Read the model definition and answer for the solid it produces. Units are mm, in the model's axes. A direction names the side the tool comes from. Round coordinates to 2 decimals unless told otherwise and drop trailing zeros. Order: outer loops, then holes, each group sorted by start corner. A loop starts at its lowest first (then second) coordinate and runs counter-clockwise, first axis right, second up. Notation, with made-up numbers: (11.25, 30.25) -> (52.25, 30.25) arc R32 cw to (52.25, 58.25) -> close; hole circle Ø11 at (18.25, 66.25). An arc over 180 degrees is marked (long way). Answer as a JSON object with one key per item and string values. Group by question number.
Item 1: Section B-B, the plane y = 26 is taken. Write down the section's boundary in (x, z), plus the area to 3 significant figures.
Item 2: Consider probe 1 along X at (y, z) = (96, 0); probe 2 along Z at (x, y) = (16, 57); probe 3 along X at (y, z) = (99, 0) (3 decimals). Determine where each line is inside the solid, lowest interval first. Write a range as from..to.
Item 3: Section C-C, the plane y = 7 is taken. Write down the section's boundary in (x, z) (3 decimals).
Item 4: Given P1, Ø5, axis at x = 8, y = 11, coming from the +Z side; P2, Ø1.3, axis at x = -11.5, y = 99, coming from the +Z side; P3, Ø0.6, axis at x = -11.5, z = 0, coming from the -Y side, each flat-ended and moving along its own axis, determine where each tip first touches the part or whether it passes through.
Item 5: The mould has two halves that part along Y. Classify faces 1 (the flat face through (5, 100, 10)), 2 (the flat face through (0, 92.5, 0)), 3 (the flat face through (-12, 99, 0)): pulls with the +Y half, pulls with the -Y half, needs draft (parallel to the pull), parting line crosses it, or undercut.
Item 6: For faces 4 (the flat face through (18.5, 0, 20.6)), 5 (the cylindrical face through (-10.74, 97.54, -2.38)), 6 (the cylindrical face through (-12.258, 93.079, -0.418)), determine the directions among +Z, -Z, +X, -X, +Y, -Y from which every point of the face is accessible in a straight line to the end or side of a thin tool.
Item 7: Section A-A, the plane x = 0 is taken. Write down the section's boundary in (y, z), plus the area to 3 significant figures.
from build123d import *

# Parameters (mm, degrees)
SKETCH2_R          = 12.5
SKETCH1_R          = 30
SKETCH5_R          = 11
CUT_EXTRUDE2_DEPTH = 5
SKETCH7_W          = 4
SKETCH7_H          = 3
CUT_EXTRUDE4_DEPTH = 12
SKETCH8_R          = 1
CUT_EXTRUDE6_DEPTH = 106.854123131
CHAMFER1_SIZE      = 2
CHAMFER1_SIZE2     = 2.698735062


# Read off the part's stored shape, not the designer's step: Shell2
with BuildPart() as part:
    # Sketch2 → Loft1 section 0
    with BuildSketch(Plane(origin=(0, 100, 0), x_dir=(1, 0, 0), z_dir=(0, 1, 0))):
        Circle(SKETCH2_R)
    # Sketch1 → Loft1 section 1
    with BuildSketch(Plane(origin=(0, 0, 0), x_dir=(1, 0, 0), z_dir=(0, 1, 0))):
        Circle(SKETCH1_R)
    loft()

    # Sketch5 → Cut-Extrude2 (cut)
    with BuildSketch(Plane(origin=(0, 100, 0), x_dir=(1, 0, 0), z_dir=(0, 1, 0))):
        with Locations(Location((0, 0, 0), (0, 0, 270))):
            Circle(SKETCH5_R)
    extrude(amount=-CUT_EXTRUDE2_DEPTH, mode=Mode.SUBTRACT)

    # Sketch7 → Cut-Extrude4 (cut)
    with BuildSketch(Plane(origin=(0, 0, 0), x_dir=(0, 0, -1), z_dir=(1, 0, 0))):
        with Locations((-0.000948901, 98.479870862)):
            Rectangle(SKETCH7_W, SKETCH7_H)
    extrude(amount=-CUT_EXTRUDE4_DEPTH, mode=Mode.SUBTRACT)

    # Shell2 outline → Shell2 (revolve, cut)
    with BuildSketch(Plane.XY):
        Polygon((11.274507437, 92.5), (0, 92.5), (0, 0), (27.462007437, 0), align=None)
    revolve(axis=Axis((0, 0, 0), (0, 1, 0)), mode=Mode.SUBTRACT)

    # Sketch8 → Cut-Extrude6 (cut, through all)
    with BuildSketch(Plane(origin=(0, 96.979870862, 0), x_dir=(1, 0, 0), z_dir=(0, 1, 0))):
        with Locations(Location((-11.275969927, 0.228612613, 0), (0, 0, 271.596209632))):
            Circle(SKETCH8_R)
    extrude(amount=-CUT_EXTRUDE6_DEPTH, mode=Mode.SUBTRACT)

    # Chamfer1
    chamfer1_edges = [part.edges().sort_by_distance(p)[0] for p in [
        (-30, 0, 0),
    ]]
    chamfer1_side = [part.faces().sort_by_distance(p)[0] for p in [
        (-29.151471863, 0, 0),
    ]]
    chamfer(chamfer1_edges, length=CHAMFER1_SIZE, length2=CHAMFER1_SIZE2, reference=chamfer1_side[0])


solid = part.part
Values found:
{
 "1": {"outline": "circle Ø50.9 at (0, 0); hole circle Ø45.82 at (0, 0)", "area": "386 mm2"},
 "2": {"probe 1": "-13.2..-12.25, 11..13.2", "probe 2": "-12.04..-7.06, 7.06..12.04", "probe 3": "-12.675..-12, 11..12.675"},
 "3": {"outline": "circle Ø57.55 at (0, 0); hole circle Ø52.474 at (0, 0)"},
 "4": {"P1": "z = 27.7", "P2": "z = 6.57", "P3": "y = 99.98"},
 "5": {"face 1": "pulls with the +Y half", "face 2": "pulls with the -Y half", "face 3": "undercut"},
 "6": {"face 4": "+Z, -Z, +X, -X, -Y", "face 5": "+Y", "face 6": "-Y"},
 "7": {"outline": "(0, -28) -> (2.66, -29.53) -> (100, -12.5) -> (100, -11) -> (95, -11) -> (95, 11) -> (100, 11) -> (100, 12.5) -> (2.66, 29.53) -> (0, 28) -> (0, 27.46) -> (92.5, 11.27) -> (92.5, -11.27) -> (0, -27.46) -> close", "area": "552 mm2"}
}
